Source: CAD feature listing. Evaluate the final solid. Frame: model axes, mm. Face numbers are marked on the shaded views. A direction names the side the tool comes from. Coordinates: 2 decimals unless noted, no trailing zeros. Loops run counter-clockwise (first coordinate to the right, second up) from the corner with the lowest first, then second, coordinate; pieces in that order, holes last. Notation, with made-up numbers: M 5,44 L 16,44 A21 cw 16,57 Z; hole C 34,66 d9. An arc over 180 degrees is marked long. One line per question, with ' | ' between items. Start each with the question number.
1. Section query A-A, the plane y = 7.75. Output: boundary loops of the cut face in (x, z).
2. Section query D-D, the plane z = 5.5. Output: boundary loops of the cut face in (x, y), and give its area (3 significant figures).
3. Mould query, pull axis X, two halves, no side actions, for the marked faces 1, 2, 3 and 4. Classes: pulls with the +X half, pulls with the -X half, needs draft (parallel to the pull), parting line crosses it, or undercut.
4. Pin query (flat end, axial travel): P1, Ø3, axis at y = 8, z = 4.5, coming from the +X side; P2, Ø5.5, axis at x = 5.883, y = 5.375, coming from the +Z side; P3, Ø1.5, axis at x = 2.5, z = 9, coming from the -Y side (3 decimals). Return the tip coordinate at first contact, or that it passes through.
5. Section query B-B, the plane y = 4.5. Output: boundary loops of the cut face in (x, z).
6. Ray query, probe 1 along X at (y, z) = (3.75, 4.25); probe 2 along Z at (x, y) = (-0.75, 5). Return the intervals inside material, ascending.
7. Access query for the marked faces 5 and 6. Directions: +Z, -Z, +X, -X, +Y, -Y. A direction counts if a zero-diameter tool reaches every point of the face in a straight line with its end or side. Return the directions, or none.
8. Section query C-C, the plane x = 4.5. Output: boundary loops of the cut face in (y, z).
```python
from build123d import *

# Parameters (mm, degrees)
SKETCH1_W                      = 10.75
SKETCH1_H                      = 10.75
BASE_FLANGE1_DEPTH             = 1.75
EDGE_FLANGE1_STRIP_W           = 9.032
EDGE_FLANGE1_STRIP_H           = 1.75
EDGE_FLANGE1_STRIP_CUT_DEPTH   = 10.75
EDGE_FLANGE1_DEPTH             = 10.75
M3_CLEARANCE_HOLE1_D           = 3.4
M3_CLEARANCE_HOLE1_ON_FACE_2_D = 3.4
FILLET1_R                      = 2


# Sheet-metal steps are written as plain solids
with BuildPart() as part:
    # Sketch1 → Base-Flange1 (new body)
    with BuildSketch(Plane.XY):
        with Locations((5.375, 5.375)):
            Rectangle(SKETCH1_W, SKETCH1_H)
    extrude(amount=-BASE_FLANGE1_DEPTH)

    # Edge-Flange1 strip (across the edge) → Edge-Flange1 strip cut (cut)
    with BuildSketch(Plane.XZ.offset(-10.75)):
        with Locations((-3.5, -0.875)):
            Rectangle(EDGE_FLANGE1_STRIP_W, EDGE_FLANGE1_STRIP_H)
    extrude(amount=EDGE_FLANGE1_STRIP_CUT_DEPTH, mode=Mode.SUBTRACT)

    # Edge-Flange1 section (across the edge) → Edge-Flange1 (add)
    with BuildSketch(Plane.XZ.offset(-10.75)):
        with BuildLine():
            Line((-1.75, 1.016), (-1.75, 10.75))
            Line((-1.75, 10.75), (0, 10.75))
            Line((0, 10.75), (0, 1.016))
            ThreePointArc((0, 1.016), (0.29757951, 0.29757951), (1.016, 0))
            Line((1.016, 0), (1.016, -1.75))
            ThreePointArc((1.016, -1.75), (-0.939857357, -0.939857357), (-1.75, 1.016))
        make_face()
    extrude(amount=EDGE_FLANGE1_DEPTH)

    # M3 Clearance Hole1 (through all)
    with Locations(Plane(origin=(5.883, 5.375, -1.75), x_dir=(-1, 0, 0), z_dir=(0, 0, -1))):
        with Locations((0, 0)):
            Hole(M3_CLEARANCE_HOLE1_D / 2)

    # M3 Clearance Hole1 on face 2 (through all)
    with Locations(Plane(origin=(-1.75, 5.375, 5.883), x_dir=(0, 0, -1), z_dir=(-1, 0, 0))):
        with Locations((0, 0)):
            Hole(M3_CLEARANCE_HOLE1_ON_FACE_2_D / 2)

    # Fillet1
    fillet1_edges = [part.edges().sort_by_distance(p)[0] for p in [
        (-0.875, 10.75, 10.75),
        (-0.875, 0, 10.75),
        (10.75, 10.75, -0.875),
        (10.75, 0, -0.875),
    ]]
    fillet(fillet1_edges, radius=FILLET1_R)


solid = part.part
```
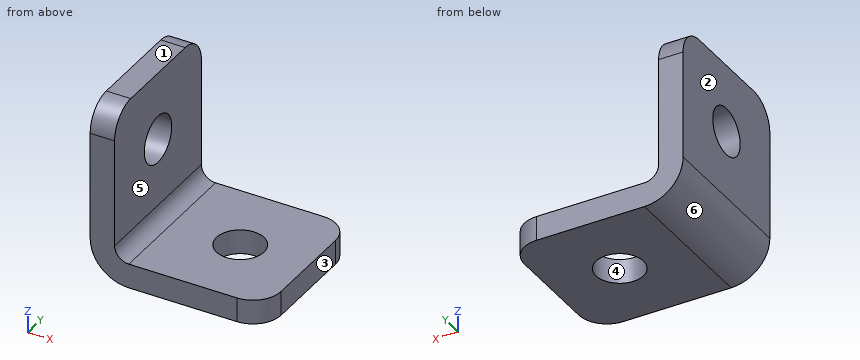
Taken from the geometry:
1) outline: M -1.75,1.02 A2.77 ccw 1.02,-1.75 L 10.75,-1.75 L 10.75,0 L 1.02,0 A1.02 cw 0,1.02 L 0,10.75 L -1.75,10.75 Z
2) outline: M -1.75,0 L 0,0 L 0,3.72 L -1.75,3.72 Z; M -1.75,7.03 L 0,7.03 L 0,10.75 L -1.75,10.75 Z | area: 13.0 mm^2
3) face 1: needs draft | face 2: pulls with the -X half | face 3: pulls with the +X half | face 4: undercut
4) P1: x = 0 | P2: z = 0 | P3: through
5) outline: M -1.75,1.02 A2.77 ccw 1.02,-1.75 L 4.43,-1.75 L 4.43,0 L 1.02,0 A1.02 cw 0,1.02 L 0,4.43 L -1.75,4.43 Z; M -1.75,7.34 L 0,7.34 L 0,10.75 L -1.75,10.75 Z; M 7.34,-1.75 L 10.75,-1.75 L 10.75,0 L 7.34,0 Z
6) probe 1: -1.75 to 0 | probe 2: -1.11 to 4.22, 7.54 to 10.75
7) face 5: +Z, +X, +Y, -Y | face 6: -Z, -X, +Y, -Y
8) outline: M 0,-1.75 L 4.39,-1.75 L 4.39,0 L 0,0 Z; M 6.36,-1.75 L 10.75,-1.75 L 10.75,0 L 6.36,0 Z
